Here's how the part is built. I have some questions about the finished solid (model axes, mm). A direction names the side the tool comes from. Coordinates: 2 decimals unless noted, no trailing zeros. Write each loop counter-clockwise with the first axis right and the second up, starting at its lowest first coordinate (ties: lowest second). Pieces come first, ordered by that corner, then holes. Notation, with made-up numbers: (84, 75) - (140, 75) arc R19 cw to (140, 94) - close; hole circle Ø10 at (-35.5, -23.5). An arc over 180 degrees is marked (long way). Answer in a Markdown table with one row per item. Add a question column.
Item 1: Imagine slicing it at C-C (x = 5). Please give me the cut outline in (y, z) (3 decimals), plus the area to 3 significant figures.
Item 2: I'm going to push flat-ended pins straight in: pin 1 (1.5 mm diameter, centred on x = 4.5, z = -10, fed in from +Y) (3 decimals); pin 2 (10 mm diameter, centred on y = 5.5, z = 5, fed in from -X); pin 3 (3.5 mm diameter, centred on y = -1.25, z = -9.1, fed in from +X); pin 4 (2.5 mm diameter, centred on y = -14, z = -9, fed in from +X). Where does each tip first touch, or does it pass through?
Item 3: Imagine slicing it at D-D (z = 18). Please give me the cut outline in (x, y) (3 decimals).
Item 4: Imagine slicing it at A-A (x = 14). State how many separate pieces and enclosed holes the cut face has, plus the area to 3 significant figures.
Item 5: Imagine slicing it at B-B (y = -1.25). Please give me the cut outline in (x, z).
Item 6: If I drill on probe 1 along Y at (x, z) = (7.5, 4.5) (3 decimals); probe 2 along Z at (x, y) = (4.05, -1.25); probe 3 along X at (y, z) = (-6, 17), over which ranges is the centre line in solid material (lowest first)? Write a range as from..to.
Item 7: Which directions (+Z, -Z, +X, -X, +Y, -Y) give clear straight access to the entire face, cutting with the end or side of a thin tool? Please do faces 1 (the face through (11, -15, -7.104)), 2 (the face through (16.04, -13.19, 7.38)), 3 (the face through (11, 13, -7.104)).
Item 8: We'd pull the mould along Z, two halves only. Please class faces 4 (the face through (3.5, -15.2, -8.5)), 5 (the face through (1.726, 12.326, -12.215)), 6 (the face through (11.105, 15.68, 22.794)): +Z half, -Z half, draft (parallel to the pull), parting line (faces both ways), or undercut.
Autodesk Inventor part; units mm, degrees
ref_plane "YZ Plane" through (0, 0, 0) normal (1, 0, 0) x (0, 1, 0)
ref_plane "XZ Plane" through (0, 0, 0) normal (0, 1, 0) x (-1, 0, 0)
ref_plane "XY Plane" through (0, 0, 0) normal (0, 0, 1) x (1, 0, 0)
sketch "Sketch1" plane through (0, 16.25, -25.5) normal (1, 0, 0) x (0, 1, 0)
  line L0 (-35, 11.3959) -> (0, 11.3959)
  line L1 (0, 11.3959) -> (0, 48.8959)
  line L2 (0, 48.8959) -> (-35, 48.8959)
  line L3 (-35, 48.8959) -> (-35, 11.3959)
  line L4 (-17.5, 1.3959) -> (0, 1.3959)
  line L5 (-35, 48.8959) -> (0, 11.3959) construction
  line L6 (-35, 11.3959) -> (0, 48.8959) construction
  line L7 (-17.5, 53) -> (-17.5, 1.3959)
  circle A0 centre (-17.5, 16.3959) radius 2
  line L8 (-35, 30.1459) -> (0, 30.1459)
  line L9 (0, 30.1459) -> (0, 48.8959)
  line L10 (0, 48.8959) -> (-35, 48.8959)
  line L11 (-35, 48.8959) -> (-35, 30.1459)
  line L12 (-35, 11.3959) -> (-27.575, 11.3959)
  line L13 (-27.575, 11.3959) -> (-27.575, 48.8959)
  line L14 (-27.575, 48.8959) -> (-35, 48.8959)
  line L15 (-35, 48.8959) -> (-35, 11.3959)
  line L16 (0, 11.3959) -> (-7.425, 11.3959)
  line L17 (-7.425, 11.3959) -> (-7.425, 48.8959)
  line L18 (-7.425, 48.8959) -> (0, 48.8959)
  line L19 (0, 48.8959) -> (0, 11.3959)
  line L20 (0, 1.3959) -> (0, 49)
  line L21 (0, 31.3959) -> (0, 11.3959)
  line L22 (0, 11.3959) -> (0, 11.3959)
  line L23 (0, 11.3959) -> (0, 48.8959)
  line L24 (-35, 20.8959) -> (0, 20.8959)
  line L25 (-35, 18.3959) -> (-27.575, 18.3959)
  line L26 (-7.425, 18.3959) -> (0, 18.3959)
  line L27 (-35, 18.3959) -> (-27.575, 11.3959) construction
  line L28 (-35, 11.3959) -> (-27.575, 18.3959) construction
  circle A1 centre (-31.2875, 14.8959) radius 1.625
  line L29 (-7.425, 11.3959) -> (0, 18.3959) construction
  line L30 (0, 11.3959) -> (-7.425, 18.3959) construction
  circle A2 centre (-3.7125, 14.8959) radius 1.625
  line L31 (-35, 48.8959) -> (-27.575, 48.8959)
  line L32 (-27.575, 48.8959) -> (-27.575, 56.3959)
  line L33 (-27.575, 56.3959) -> (-35, 56.3959)
  line L34 (-35, 56.3959) -> (-35, 48.8959)
  line L35 (0, 48.8959) -> (-7.425, 48.8959)
  line L36 (-7.425, 48.8959) -> (-7.425, 56.3959)
  line L37 (-7.425, 56.3959) -> (0, 56.3959)
  line L38 (0, 56.3959) -> (0, 48.8959)
  line L39 (-35, 48.8959) -> (-27.575, 56.3959) construction
  line L40 (-35, 56.3959) -> (-27.575, 48.8959) construction
  line L41 (-7.425, 48.8959) -> (0, 56.3959) construction
  line L42 (-7.425, 56.3959) -> (0, 48.8959) construction
  circle A3 centre (-3.7125, 52.6459) radius 1.625
  circle A4 centre (-31.2875, 52.6459) radius 1.625
  circle A5 centre (-31.2875, 33.6459) radius 2
  circle A6 centre (-3.7125, 33.6459) radius 2
  line L43 (-27.575, 18.3959) -> (-35, 48.8959) construction
  line L44 (-35, 18.3959) -> (-27.575, 48.8959) construction
  line L45 (-27.575, 48.8959) -> (-7.425, 48.8959)
  line L46 (-7.425, 48.8959) -> (-7.425, 56.3959)
  line L47 (-7.425, 56.3959) -> (-27.575, 56.3959)
  line L48 (-27.575, 56.3959) -> (-27.575, 48.8959)
  point P0 (-17.5, 48.8959)
  point P1 (-17.5, 30.1459)
  point P2 (-1.25, 11.3959)
  point P3 (-27.575, 48.8959)
  point P4 (-27.575, 30.1459)
  point P5 (-7.425, 30.1459)
  point P6 (-7.425, 48.8959)
  point P7 (-7.425, 11.3959)
  point P8 (-27.575, 11.3959)
  point P9 (-17.5, 48.8959)
  point P10 (-17.5, 11.3959)
  point P11 (-1.25, 11.3959)
  point P12 (-7.425, 20.8959)
  point P13 (-27.575, 20.8959)
  point P14 (0, 20.8959)
  point P15 (-35, 20.8959)
  point P16 (-35, 18.3959)
  point P17 (0, 18.3959)
  point P18 (0, 48.8959)
  point P19 (-7.425, 48.8959)
  point P20 (0, 48.8959)
  point P21 (-3.7125, 14.8959)
  point P22 (-27.575, 48.8959)
  point P23 (-7.425, 48.8959)
  point P24 (0, 11.3959)
  point P25 (0, 48.8959)
  dimension "d5" = 37.5
  dimension "d3" = 10
  dimension "d4" = 35
  dimension "d2" = 4
  dimension "d18" = 5
  dimension "d19" = 4.5
  dimension "d20" = 2.5
  dimension "d21" = 3.25
  dimension "d23" = 7.5
  dimension "d24" = 4
  dimension "d25" = 4
  dimension "d29" = 7.5
  dimension "d30" = 20.15
extrude "Extrusion1" add sketch "Sketch1" along normal blind 2 contours L3 L25 L13 L0 | L13 L24 L7 A0 L0 | L3 L24 L13 L25 | L7 A0 L24 L17 L0 | L3 L8 L13 L24 | L17 L26 L1 L0 | A0 L7 | L7 A0 | L13 L8 L7 L24 | L3 L2 L13 L8 | L17 L24 L1 L26 | L13 L2 L7 L8 | L7 L8 L17 L24 | L34 L33 L32 L2 | L17 L8 L1 L24 | L7 L2 L17 L8 | L32 L47 L36 L2 | L17 L2 L1 L8 | L36 L37 L38 L20 L2 | A5 | A6
extrude "Extrusion2" add sketch "Sketch1" along normal blind 1.5 from surface at 2 contours L3 L25 L13 L0 | L13 L24 L7 A0 L0 | L3 L24 L13 L25 | L7 A0 L24 L17 L0 | L3 L8 L13 L24 | L17 L26 L1 L0 | L13 L8 L7 L24 | L3 L2 L13 L8 | L17 L24 L1 L26 | L13 L2 L7 L8 | L7 L8 L17 L24 | L34 L33 L32 L2 | L17 L8 L1 L24 | L7 L2 L17 L8 | L32 L47 L36 L2 | L17 L2 L1 L8 | L36 L37 L38 L20 L2 | A5 | A6
extrude "Extrusion3" add sketch "Sketch1" along normal blind 3.5 from surface at 3.5 contours L13 L24 L7 A0 L0 | L7 A0 L24 L17 L0
extrude "Extrusion4" add sketch "Sketch1" along normal blind 15 from surface at 3.5 contours L3 L24 L13 L25 | L3 L8 L13 L24 | L3 L2 L13 L8 | L17 L24 L1 L26 | L17 L8 L1 L24 | L17 L2 L1 L8 | A5 | A6
fillet "Fillet1" radius 2 16 edges at (1.75, -18.75, -14.1041) (11, -18.75, -7.1041) (5.25, -11.325, -7.1041) (12.75, -11.325, -7.1041) (5.25, -11.325, -14.1041) (5.25, 8.825, -14.1041) (5.25, 8.825, -7.1041) (12.75, 8.825, -7.1041) (11, 16.25, -7.1041) (11, -11.325, 23.3959) (11, 8.825, 23.3959) (1.75, -18.75, 30.8959) (11, -18.75, 23.3959) (11, 16.25, 23.3959) (1.75, 16.25, 30.8959) (1.75, 16.25, -14.1041)
extrude "Extrusion5" cut sketch "Sketch1" against normal blind 5 from surface at 18.5 contours A5 | A6
properties part number "MotorMount"
Here are the results:
| question | item | result |
|---|---|---|
| 1 | outline | (-18.75, -5.104) arc R2 ccw to (-16.75, -7.104) - (-13.325, -7.104) arc R2 cw to (-11.325, -9.104) - (-11.325, -12.104) arc R2 ccw to (-9.325, -14.104) - (6.825, -14.104) arc R2 ccw to (8.825, -12.104) - (8.825, -9.104) arc R2 cw to (10.825, -7.104) - (14.25, -7.104) arc R2 ccw to (16.25, -5.104) - (16.25, 21.396) arc R2 ccw to (14.25, 23.396) - (10.825, 23.396) arc R2 ccw to (8.825, 21.396) - (8.825, -4.604) - (-11.325, -4.604) - (-11.325, 21.396) arc R2 ccw to (-13.325, 23.396) - (-16.75, 23.396) arc R2 ccw to (-18.75, 21.396) - close; hole circle Ø4 at (-1.25, -9.104) |
| 1 | area | 627 mm2 |
| 2 | pin 1 | stops at y = 8.825 |
| 2 | pin 2 | stops at x = 0 |
| 2 | pin 3 | stops at x = 2 |
| 2 | pin 4 | stops at x = 3.5 |
| 3 | outline | (0, -18.75) - (18.5, -18.75) - (18.5, -11.325) - (3.5, -11.325) - (3.5, 8.825) - (18.5, 8.825) - (18.5, 16.25) - (0, 16.25) - close |
| 4 | separate pieces | 2 |
| 4 | enclosed holes | 2 |
| 4 | area | 421 mm2 |
| 5 | outline | (0, -14.1) - (7, -14.1) - (7, -11.1) - (2, -11.1) - (2, -7.1) - (7, -7.1) - (7, -4.6) - (3.5, -4.6) - (3.5, 30.9) - (0, 30.9) - close |
| 6 | probe 1 | y = -18.75..-11.325, 8.825..16.25 |
| 6 | probe 2 | z = -14.1..-11.1, -7.1..-4.6 |
| 6 | probe 3 | x = 0..3.5 |
| 7 | face 1 | -Z, +X, -Y |
| 7 | face 2 | +X |
| 7 | face 3 | -Z, +X, +Y |
| 8 | face 4 | draft |
| 8 | face 5 | undercut |
| 8 | face 6 | +Z half |
